Could you check a few things on this drawing? It's one solid part, dimensions in mm from its lowest x, y, z. Give positions to 0.01 mm unless a question says otherwise; leave off trailing zeros. Loops run counter-clockwise (first coordinate to the right, second up) from the corner with the lowest first, then second, coordinate; pieces in that order, holes last. Notation, with made-up numbers: (30, -28.75) -> (42, -28.75) arc R26 cw to (42, 3.25) -> close; hole circle Ø1 at (58, 86). An arc over 180 degrees is marked (long way). Use CSV: the item, a comma, the result in double quotes.
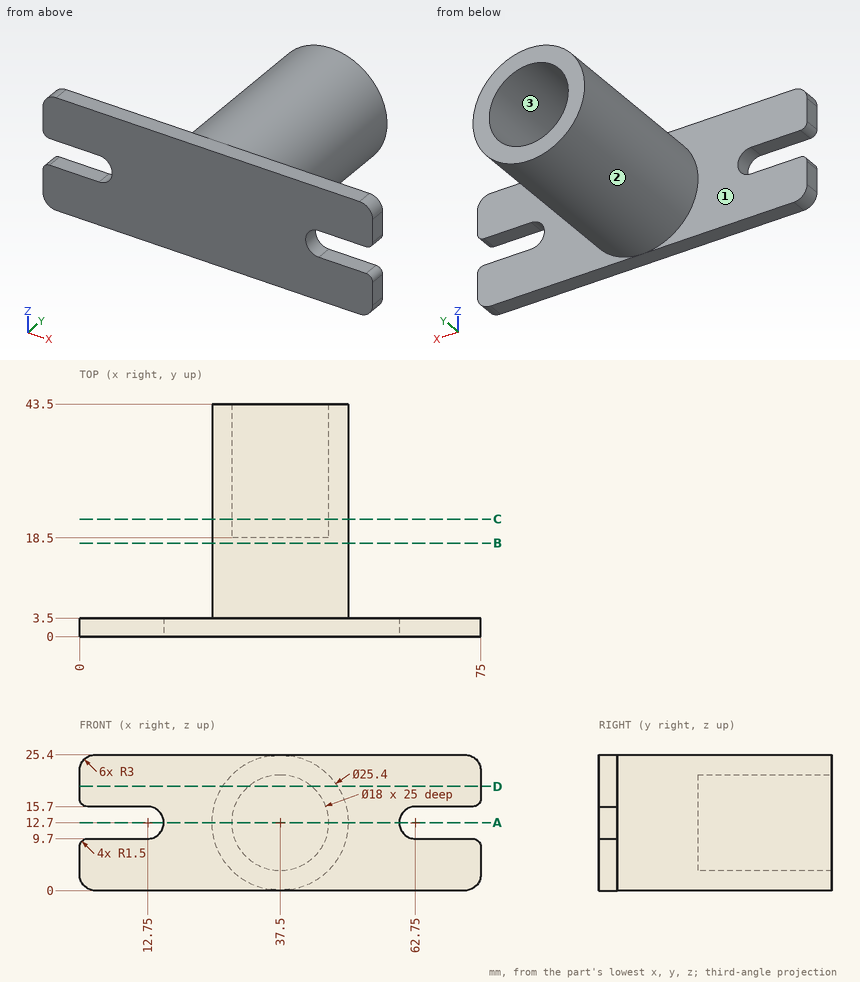
(1) If we section it at B-B, the plane y = 17.5: Write out the boundary of the cut face in (x, z), then the cut area to 3 significant figures.
Answer sheet:
outline,"circle Ø25.4 at (37.5, 12.7)"
area,"507 mm2"
(2) If I drill on L1, parallel to X at y = 38, z = 12.7; L2, parallel to Y at x = 40.5, z = 21; L3, parallel to Y at x = 64.5, z = 23, over which ranges is the centre line in solid material (lowest first)? Write a range as from..to.
Answer sheet:
L1,"x = 24.8..28.5, 46.5..50.2"
L2,"y = 0..18.5"
L3,"y = 0..3.5"
(3) Will these pins go through, and if not, where does the flat tip stop? pin 1 Ø3 at (y, z) = (14, 13) entering from -X; pin 2 Ø8 at (y, z) = (19.5, 19) entering from -X; pin 3 Ø9 at (x, z) = (40.5, 12.5) entering from +Y.
Answer sheet:
pin 1,"stops at x = 24.8"
pin 2,"stops at x = 25.01"
pin 3,"stops at y = 18.5"
(4) We'd pull the mould along X, two halves only. Please class the marked faces 1, 2 and 3: released by +X, released by -X, zero draft, split by the parting line, or undercut.
Answer sheet:
face 1,"zero draft"
face 2,"split by the parting line"
face 3,"undercut"
(5) If we section it at A-A, the plane z = 12.7: Write out the boundary of the cut face in (x, y), then the cut area to 3 significant figures.
Answer sheet:
outline,"(15.75, 0) -> (59.75, 0) -> (59.75, 3.5) -> (50.2, 3.5) -> (50.2, 43.5) -> (46.5, 43.5) -> (46.5, 18.5) -> (28.5, 18.5) -> (28.5, 43.5) -> (24.8, 43.5) -> (24.8, 3.5) -> (15.75, 3.5) -> close"
area,"720 mm2"
(6) If we section it at C-C, the plane y = 22: Write out the boundary of the cut face in (x, z), then the cut area to 3 significant figures.
Answer sheet:
outline,"circle Ø25.4 at (37.5, 12.7); hole circle Ø18 at (37.5, 12.7)"
area,"252 mm2"
(7) If we section it at D-D, the plane z = 19.5: Write out the boundary of the cut face in (x, y).
Answer sheet:
outline,"(0, 0) -> (75, 0) -> (75, 3.5) -> (48.23, 3.5) -> (48.23, 43.5) -> (43.4, 43.5) -> (43.4, 18.5) -> (31.6, 18.5) -> (31.6, 43.5) -> (26.77, 43.5) -> (26.77, 3.5) -> (0, 3.5) -> close"
